Geometry check sheet. Reference: the model listing, model coordinates, mm. Face numbers are marked on the shaded views. Give positions to 0.01 mm unless a question says otherwise; leave off trailing zeros. Loops run counter-clockwise (first coordinate to the right, second up) from the corner with the lowest first, then second, coordinate; pieces in that order, holes last. Notation, with made-up numbers: (17.25, -32.75) -> (41.25, -32.75) arc R21 ccw to (41.25, -11.75) -> close; hole circle Ø1 at (49, 86.5). An arc over 180 degrees is marked (long way). Write each question's results on one line, items separated by ' | '. Start each with the question number.
1) Depth check by flat-ended pin: pin 1 (6 mm diameter, centred on y = 12.5, z = 7.5, fed in from -X); pin 2 (6 mm diameter, centred on x = 24.5, y = 11, fed in from +Z); pin 3 (3 mm diameter, centred on y = 28.5, z = 4, fed in from -X); pin 4 (0.6 mm diameter, centred on y = 22, z = 1.5, fed in from -X). Enter the tip coordinate at first touch or a pass-through.
2) Draft check along X on the marked faces 1 and 2. Enter one of: pulls with the +X half, pulls with the -X half, needs draft (parallel to the pull), parting line crosses it, or undercut.
3) Sectioned sample at B-B on x = 32. Record the cut outline in (y, z).
4) Scan lines: line 1 (Y direction, x = 3, z = 25.8); line 2 (Y direction, x = 3, z = 27.05); line 3 (Z direction, x = 36.5, y = 7.5). Record each from-to range of solid material in increasing order. Write a range as from..to.
5) Sectioned sample at A-A on z = 14.25. Record the cut outline in (x, y), then the cut area to 3 significant figures.
```python
from build123d import *

# Parameters (mm, degrees)
PAD_DEPTH       = 2
SKETCH001_R     = 2
PAD001_DEPTH    = 25
SKETCH002_R     = 1.5
PAD002_DEPTH    = 2
SKETCH003_R     = 1.5
PAD003_DEPTH    = 2
SKETCH004_R     = 0.5
POCKET_DEPTH    = 5
SKETCH005_R     = 0.5
POCKET001_DEPTH = 5


with BuildPart() as part:
    # Sketch → Pad (new body)
    with BuildSketch(Plane.XY):
        Polygon((0, 39), (54, 39), (54, 0), (0, 0), (0, 16.5), (3, 16.5), (3, 26.5), (0, 26.5), align=None)
    extrude(amount=PAD_DEPTH)

    # Sketch001 (on Face10 of Pad) → Pad001 (join)
    with BuildSketch(Plane.XY.offset(2)):
        with Locations((3, 14)):
            Circle(SKETCH001_R)
        with Locations((51, 14)):
            Circle(SKETCH001_R)
    extrude(amount=PAD001_DEPTH)

    # Sketch002 (on Face13 of Pad001) → Pad002 (join)
    with BuildSketch(Plane.XY.offset(27)):
        with Locations((3, 14)):
            Circle(SKETCH002_R)
    extrude(amount=PAD002_DEPTH)

    # Sketch003 (on Face14 of Pad002) → Pad003 (join)
    with BuildSketch(Plane.XY.offset(27)):
        with Locations((51, 14)):
            Circle(SKETCH003_R)
    extrude(amount=PAD003_DEPTH)

    # Sketch004 (on Face17 of Pad003) → Pocket (cut)
    with BuildSketch(Plane.XY.offset(29)):
        with Locations((3, 14)):
            Circle(SKETCH004_R)
    extrude(amount=-POCKET_DEPTH, mode=Mode.SUBTRACT)

    # Sketch005 (on Face18 of Pocket) → Pocket001 (cut)
    with BuildSketch(Plane.XY.offset(29)):
        with Locations((51, 14)):
            Circle(SKETCH005_R)
    extrude(amount=-POCKET001_DEPTH, mode=Mode.SUBTRACT)


solid = part.part
```
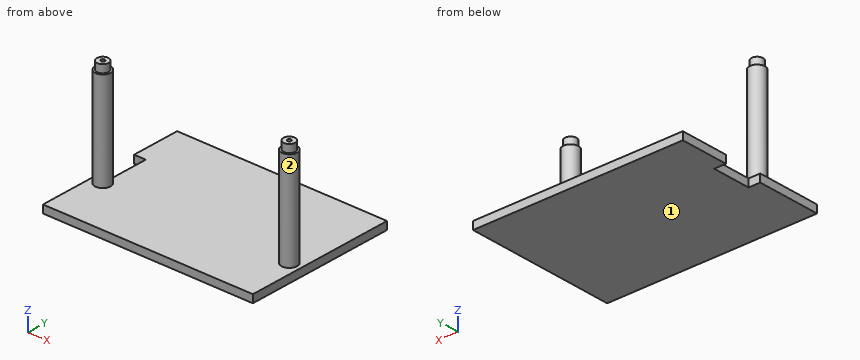
Result:
1) pin 1: x = 1 | pin 2: z = 2 | pin 3: through | pin 4: x = 3
2) face 1: needs draft | face 2: undercut
3) outline: (0, 0) -> (39, 0) -> (39, 2) -> (0, 2) -> close
4) line 1: 12..13.5, 14.5..16 | line 2: 12.5..13.5, 14.5..15.5 | line 3: 0..2
5) outline: circle Ø4 at (3, 14); circle Ø4 at (51, 14) | area: 25.1 mm^2
